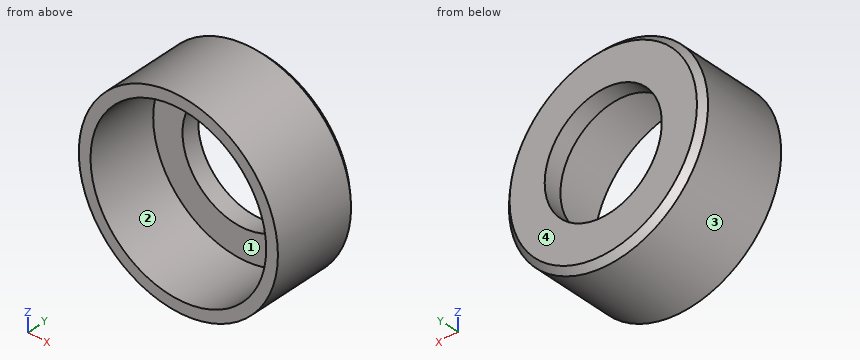
```python
from build123d import *

# Parameters (mm, degrees)
SKETCH1_R           = 8.5
SKETCH1_R_2         = 7.5
BOSS_EXTRUDE1_DEPTH = 6
SKETCH3_R           = 8.5
SKETCH3_R_2         = 5
BOSS_EXTRUDE2_DEPTH = 1.5
CHAMFER1_SIZE       = 0.5


with BuildPart() as part:
    # Sketch1 → Boss-Extrude1 (new body)
    with BuildSketch(Plane(origin=(0, 0, 0), x_dir=(1, 0, 0), z_dir=(0, 1, 0))):
        Circle(SKETCH1_R)
        Circle(SKETCH1_R_2, mode=Mode.SUBTRACT)
    extrude(amount=BOSS_EXTRUDE1_DEPTH)

    # Sketch3 → Boss-Extrude2 (add)
    with BuildSketch(Plane(origin=(0, 6, 0), x_dir=(1, 0, 0), z_dir=(0, 1, 0))):
        Circle(SKETCH3_R)
        Circle(SKETCH3_R_2, mode=Mode.SUBTRACT)
    extrude(amount=BOSS_EXTRUDE2_DEPTH)

    # Chamfer1
    chamfer1_edges = [part.edges().sort_by_distance(p)[0] for p in [
        (-8.5, 7.5, 0),
    ]]
    chamfer(chamfer1_edges, length=CHAMFER1_SIZE)


solid = part.part
```
The listing builds one solid part. Answer for the finished solid, in the listing's coordinates (mm). Face numbers are marked on the shaded views. Give positions to 0.01 mm unless a question says otherwise; leave off trailing zeros. Order: outer loops, then holes, each group sorted by start corner. A loop starts at its lowest first (then second) coordinate and runs counter-clockwise, first axis right, second up. Notation, with made-up numbers: (-3.5, 50.25) -> (53.5, 50.25) arc R21 ccw to (53.5, 89.25) -> close; hole circle Ø5 at (57.25, 81). An arc over 180 degrees is marked (long way). Answer as CSV lines item,"result". Start each with the question number.
Q1. A cutting plane is placed at B-B (x = 0). Determine the outline of the cut face in (y, z), then the cut area to 4 significant figures.
Q2. Find the intervals of material crossed by L1, parallel to Z at x = 0, y = 6.45; L2, parallel to X at y = 1.8, z = 0, in increasing order.
Q3. A cutting plane is placed at C-C (y = 3). Determine the outline of the cut face in (x, z), then the cut area to 3 significant figures.
Q4. A cutting plane is placed at A-A (z = 0). Determine the outline of the cut face in (x, y), then the cut area to 4 significant figures.
Q5. Given pin 1 (3 mm diameter, centred on y = 1.5, z = 2, fed in from -X); pin 2 (1 mm diameter, centred on x = 1.5, y = 4.5, fed in from +Z); pin 3 (1.5 mm diameter, centred on y = 3, z = -4, fed in from +X), each flat-ended and moving along its own axis, determine where each tip first touches the part or whether it passes through.
Q6. Determine the mould class of the marked faces 1, 2, 3 and 4 for opening direction Z: pulls with the +Z half, pulls with the -Z half, needs draft (parallel to the pull), parting line crosses it, or undercut.
Results found:
1,outline,"(0, -8.5) -> (7, -8.5) -> (7.5, -8) -> (7.5, -5) -> (6, -5) -> (6, -7.5) -> (0, -7.5) -> close; (0, 7.5) -> (6, 7.5) -> (6, 5) -> (7.5, 5) -> (7.5, 8) -> (7, 8.5) -> (0, 8.5) -> close"
1,area,"22.25 mm2"
2,L1,"-8.5 to -5, 5 to 8.5"
2,L2,"-8.5 to -7.5, 7.5 to 8.5"
3,outline,"circle Ø17 at (0, 0); hole circle Ø15 at (0, 0)"
3,area,"50.3 mm2"
4,outline,"(-8.5, 0) -> (-7.5, 0) -> (-7.5, 6) -> (-5, 6) -> (-5, 7.5) -> (-8, 7.5) -> (-8.5, 7) -> close; (5, 6) -> (7.5, 6) -> (7.5, 0) -> (8.5, 0) -> (8.5, 7) -> (8, 7.5) -> (5, 7.5) -> close"
4,area,"22.25 mm2"
5,pin 1,"x = -8.49"
5,pin 2,"z = 8.44"
5,pin 3,"x = 7.85"
6,face 1,"undercut"
6,face 2,"undercut"
6,face 3,"parting line crosses it"
6,face 4,"needs draft"
